```python
from build123d import *

# Parameters (mm, degrees)
F0_W     = 50.8
F0_H     = 304.8
F1_DEPTH = 1.5875
F2_W     = 114.3
F2_H     = 304.8
F3_DEPTH = 1.5875
F4_W     = 50.8
F4_H     = 304.8
F5_DEPTH = 1.5875
F6_R     = 3.175
F7_DEPTH = 136.906
F8_R     = 3.175
F9_DEPTH = 146.304


with BuildPart() as f1:
    # F0 (on Front) → F1 (new body)
    with BuildSketch(Plane.XZ):
        Rectangle(F0_W, F0_H)
    extrude(amount=-F1_DEPTH)

    # F2 (on face) → F3 (join)
    with BuildSketch(Plane(origin=(-25.4, 0, 0), x_dir=(0, -1, 0), z_dir=(-1, 0, 0))):
        with Locations((-57.15, 0)):
            Rectangle(F2_W, F2_H)
    extrude(amount=-F3_DEPTH)

    # F4 (on face) → F5 (join)
    with BuildSketch(Plane(origin=(0, 114.3, 0), x_dir=(-1, 0, 0), z_dir=(0, 1, 0))):
        Rectangle(F4_W, F4_H)
    extrude(amount=-F5_DEPTH)

    # F6 (on face) → F7 (cut)
    with BuildSketch(Plane(origin=(0, 114.3, 0), x_dir=(-1, 0, 0), z_dir=(0, 1, 0))):
        with Locations((20.58794, 148.060083)):
            Circle(F6_R)
    extrude(amount=-F7_DEPTH, mode=Mode.SUBTRACT)

    # F8 (on face) → F9 (cut)
    with BuildSketch(Plane.XZ):
        Circle(F8_R)
    extrude(amount=-F9_DEPTH, mode=Mode.SUBTRACT)


solid = f1.part
```
Geometry: final body of the model. Coordinates: model frame, mm. A direction names the side the tool comes from. Round coordinates to 2 decimals unless told otherwise and drop trailing zeros. Order: outer loops, then holes, each group sorted by start corner. A loop starts at its lowest first (then second) coordinate and runs counter-clockwise, first axis right, second up. Notation, with made-up numbers: (34.25, 11.25) - (90.25, 11.25) arc R23 cw to (90.25, 28.25) - close; hole circle Ø11 at (65, 8). An arc over 180 degrees is marked (long way). Use CSV: the item, a comma, the result in double quotes. Start each with the question number.
Q1. First-contact query: pin 1 (1 mm diameter, centred on y = 68, z = 59.5, fed in from +X). Flat tip, straight axial feed; report the tip coordinate or a pass-through.
Q2. Section query C-C (x = 0). Return loops of the section in (y, z) (1 decimal), and give its area (3 significant figures).
Q3. Section query D-D (z = 0). Return loops of the section in (x, y) (1 decimal), and give its area (3 significant figures).
Q4. Material intervals for line 1 along Y through (x, z) = (-19, -104); line 2 along Z through (x, y) = (0, 113.6) (3 decimals); line 3 along X through (y, z) = (33, -59.5), sorted ascending. Write a range as from..to.
Q5. Section query B-B (z = -109). Return loops of the section in (x, y), and give its area (3 significant figures).
Q6. Access query for faces 1 (the face through (-19.9, 113.52, 144.96)), 2 (the face through (7, 112.712, 2)). Directions: +Z, -Z, +X, -X, +Y, -Y. A direction counts if a zero-diameter tool reaches every point of the face in a straight line with its end or side. Return the directions, or none.
Q7. Mould query, pull axis Z, two halves, no side actions, for faces 3 (the face through (-24, 57, 152.4)), 4 (the face through (-0.69, 113.5, -3.1)), 5 (the face through (-25.4, 58, 2)). Classes: +Z half, -Z half, draft (parallel to the pull), parting line (faces both ways), or undercut.
Q8. Section query A-A (x = 13). Return loops of the section in (y, z).
Result set:
1,pin 1,"stops at x = -23.81"
2,outline,"(0, -152.4) - (1.6, -152.4) - (1.6, -3.2) - (0, -3.2) - close; (0, 3.2) - (1.6, 3.2) - (1.6, 152.4) - (0, 152.4) - close; (112.7, -152.4) - (114.3, -152.4) - (114.3, -3.2) - (112.7, -3.2) - close; (112.7, 3.2) - (114.3, 3.2) - (114.3, 152.4) - (112.7, 152.4) - close"
2,area,"948 mm2"
3,outline,"(-25.4, 0) - (-3.2, 0) - (-3.2, 1.6) - (-23.8, 1.6) - (-23.8, 112.7) - (-3.2, 112.7) - (-3.2, 114.3) - (-25.4, 114.3) - close; (3.2, 0) - (25.4, 0) - (25.4, 1.6) - (3.2, 1.6) - close; (3.2, 112.7) - (25.4, 112.7) - (25.4, 114.3) - (3.2, 114.3) - close"
3,area,"318 mm2"
4,line 1,"y = 0..1.59, 112.71..114.3"
4,line 2,"z = -152.4..-3.175, 3.175..152.4"
4,line 3,"x = -25.4..-23.81"
5,outline,"(-25.4, 0) - (25.4, 0) - (25.4, 1.59) - (-23.81, 1.59) - (-23.81, 112.71) - (25.4, 112.71) - (25.4, 114.3) - (-25.4, 114.3) - close"
5,area,"338 mm2"
6,face 1,"+Y, -Y"
6,face 2,"+Z, -Z, +X"
7,face 3,"+Z half"
7,face 4,"undercut"
7,face 5,"draft"
8,outline,"(0, -152.4) - (1.59, -152.4) - (1.59, 152.4) - (0, 152.4) - close; (112.71, -152.4) - (114.3, -152.4) - (114.3, 152.4) - (112.71, 152.4) - close"
